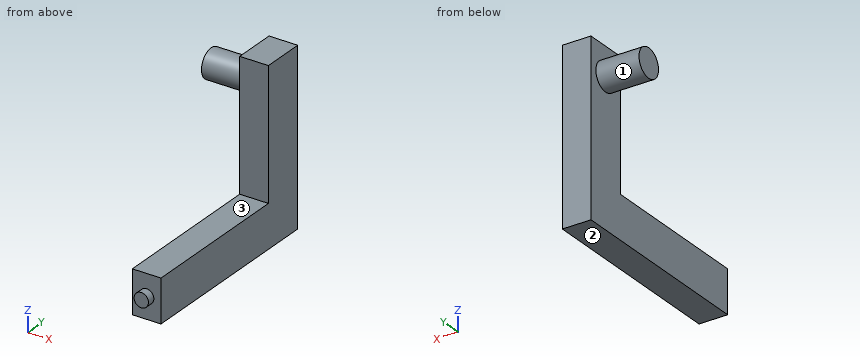
from build123d import *

# Parameters (mm, degrees)
F0_W     = 4
F0_H     = 18
F1_DEPTH = 6
F0_H_2   = 6
F2_DEPTH = 28
F3_R     = 1
F4_DEPTH = 1.1
F5_R     = 2
F6_DEPTH = 6


with BuildPart() as f1:
    # F0 (on Front) → F1 (new body)
    with BuildSketch(Plane.XZ):
        with Locations((0, 12.794577)):
            Rectangle(F0_W, F0_H)
    extrude(amount=F1_DEPTH)

    # F0 (on Front) → F2 (join)
    with BuildSketch(Plane.XZ):
        with Locations((0, 0.794577)):
            Rectangle(F0_W, F0_H_2)
    extrude(amount=F2_DEPTH)

    # F3 (on face) → F4 (join)
    with BuildSketch(Plane.XZ.offset(28)):
        with Locations((0, 0.794577)):
            Circle(F3_R)
    extrude(amount=F4_DEPTH)

    # F5 (on face) → F6 (join)
    with BuildSketch(Plane(origin=(-2, 0, 0), x_dir=(0, -1, 0), z_dir=(-1, 0, 0))):
        with Locations((3, 17.794577)):
            Circle(F5_R)
    extrude(amount=F6_DEPTH)


solid = f1.part
Read the model definition and answer for the solid it produces. Units are mm, in the model's axes. Face numbers are marked on the shaded views. A direction names the side the tool comes from. Give positions to 0.01 mm unless a question says otherwise; leave off trailing zeros. Write each loop counter-clockwise with the first axis right and the second up, starting at its lowest first coordinate (ties: lowest second). Pieces come first, ordered by that corner, then holes. Notation, with made-up numbers: (-1, 53.5) - (10, 53.5) arc R24 ccw to (10, 65.5) - close; hole circle Ø3 at (40, 30.5). An arc over 180 degrees is marked (long way). Return JSON: item names as keys, results as strings.
Q1. Consider line 1 along X through (y, z) = (-19.25, 0); line 2 along Y through (x, z) = (0, 16); line 3 along Z through (x, y) = (-1.5, -13). Determine where each line is inside the solid, lowest interval first. Write a range as [from, to].
Reply:
{"line 1": "[-2, 2]", "line 2": "[-6, 0]", "line 3": "[-2.21, 3.79]"}
Q2. For the marked faces 1, 2 and 3, determine the directions among +Z, -Z, +X, -X, +Y, -Y from which every point of the face is accessible in a straight line to the end or side of a thin tool.
Reply:
{"face 1": "-X", "face 2": "-Z, +X, -X, +Y, -Y", "face 3": "+Z, +X, -X, -Y"}
Q3. A cutting plane is placed at D-D, the plane x = 0. Determine the outline of the cut face in (y, z), and give its area (3 significant figures).
Reply:
{"outline": "(-29.1, -0.21) - (-28, -0.21) - (-28, -2.21) - (0, -2.21) - (0, 21.79) - (-6, 21.79) - (-6, 3.79) - (-28, 3.79) - (-28, 1.79) - (-29.1, 1.79) - close", "area": "278 mm²"}
Q4. Given P1, Ø1.2, axis at x = 1, y = -15, coming from the +Z side; P2, Ø1, axis at y = -20.5, z = 0.5, coming from the -X side; P3, Ø4.5, axis at x = -0.5, z = 14.5, coming from the -Y side, each flat-ended and moving along its own axis, determine where each tip first touches the part or whether it passes through.
Reply:
{"P1": "z = 3.79", "P2": "x = -2", "P3": "y = -6"}
Q5. A cutting plane is placed at B-B, the plane z = 0.25. Determine the outline of the cut face in (x, y), and give its area (3 significant figures).
Reply:
{"outline": "(-2, -28) - (-0.84, -28) - (-0.84, -29.1) - (0.84, -29.1) - (0.84, -28) - (2, -28) - (2, 0) - (-2, 0) - close", "area": "114 mm²"}
Q6. A cutting plane is placed at A-A, the plane x = -1.5. Determine the outline of the cut face in (y, z).
Reply:
{"outline": "(-28, -2.21) - (0, -2.21) - (0, 21.79) - (-6, 21.79) - (-6, 3.79) - (-28, 3.79) - close"}
Q7. A cutting plane is placed at C-C, the plane y = -3. Determine the outline of the cut face in (x, z).
Reply:
{"outline": "(-8, 15.79) - (-2, 15.79) - (-2, -2.21) - (2, -2.21) - (2, 21.79) - (-2, 21.79) - (-2, 19.79) - (-8, 19.79) - close"}
